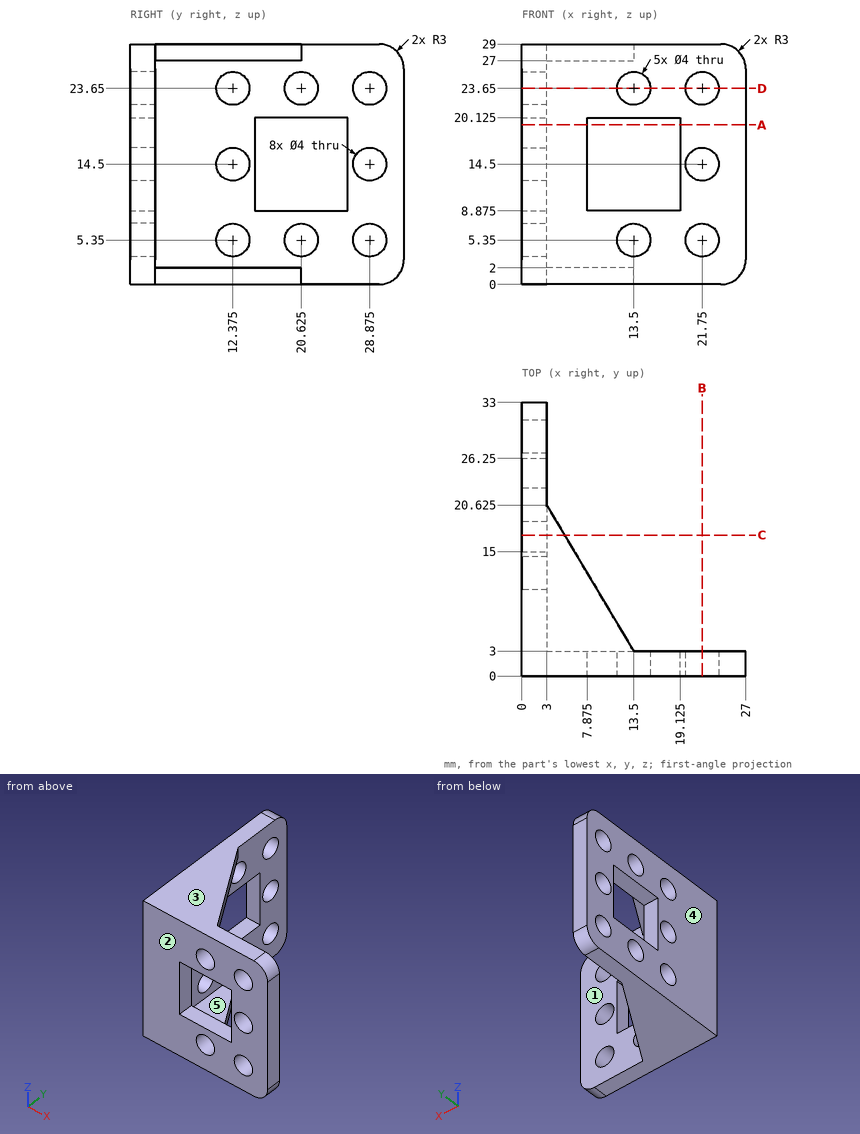
Check sheet for the drawn part. Datum: minimum x, y, z corner. Units: mm. A direction names the side the tool comes from. Round coordinates to 2 decimals unless told otherwise and drop trailing zeros. Loops run counter-clockwise (first coordinate to the right, second up) from the corner with the lowest first, then second, coordinate; pieces in that order, holes last. Notation, with made-up numbers: (24.5, -22) - (42.5, -22) arc R10 cw to (42.5, -16) - close; hole circle Ø2 at (-34.5, 42.25). An arc over 180 degrees is marked (long way). Answer as a JSON object with one key per item and string values. Group by question number.
Q1. Mould release check, pull along Z, two halves, no side actions. Record for the marked faces 3, 4 and 5: released by +Z, released by -Z, zero draft, split by the parting line, or undercut.
Q2. Sectioned sample at D-D, the plane z = 23.65. Enter the section's corners in (x, y) (3 decimals), plus the area to 3 significant figures.
Q3. Sectioned sample at A-A, the plane z = 19.25. Enter the section's corners in (x, y) (3 decimals), plus the area to 4 significant figures.
Q4. Sectioned sample at C-C, the plane y = 17. Enter the section's corners in (x, z) (3 decimals), plus the area to 3 significant figures.
Q5. Scan lines: line 1 along Z through (x, y) = (21.75, 2.2); line 2 along Y through (x, z) = (2.05, 23.65) (3 decimals); line 3 along Z through (x, y) = (13.5, 1.9) (3 decimals). Record each from-to range of solid material in increasing order. Write a range as [from, to].
Q6. Gauge pin test, flat end, axial feed: P1, Ø14.5, axis at y = 11.5, z = 19, coming from the +X side. Record the tip position at first contact, or that the pin passes through.
Q7. Sectioned sample at B-B, the plane x = 21.75. Enter the section's corners in (y, z).
Q8. Set-up check for the marked faces 1 and 2: record each of +Z, -Z, +X, -X, +Y, -Y from which the full face is reachable in a straight line by a thin tool's end or side.
Solution:
{
 "1": {"face 3": "released by +Z", "face 4": "zero draft", "face 5": "undercut"},
 "2": {"outline": "(0, 0) - (11.5, 0) - (11.5, 3) - (3, 3) - (3, 10.375) - (0, 10.375) - close; (0, 14.375) - (3, 14.375) - (3, 18.625) - (0, 18.625) - close; (0, 22.625) - (3, 22.625) - (3, 26.875) - (0, 26.875) - close; (0, 30.875) - (3, 30.875) - (3, 33) - (0, 33) - close; (15.5, 0) - (19.75, 0) - (19.75, 3) - (15.5, 3) - close; (23.75, 0) - (27, 0) - (27, 3) - (23.75, 3) - close", "area": "111 mm²"},
 "3": {"outline": "(0, 0) - (7.875, 0) - (7.875, 3) - (3, 3) - (3, 15) - (0, 15) - close; (0, 26.25) - (3, 26.25) - (3, 33) - (0, 33) - close; (19.125, 0) - (27, 0) - (27, 3) - (19.125, 3) - close", "area": "103.5 mm²"},
 "4": {"outline": "(0, 0) - (5.16, 0) - (5.16, 2) - (3, 2) - (3, 8.875) - (0, 8.875) - close; (0, 20.125) - (3, 20.125) - (3, 27) - (5.16, 27) - (5.16, 29) - (0, 29) - close", "area": "61.9 mm²"},
 "5": {"line 1": "z = [0, 3.35], [7.35, 12.5], [16.5, 21.65], [25.65, 29]", "line 2": "y = [0, 10.375], [14.375, 18.625], [22.625, 26.875], [30.875, 33]", "line 3": "z = [0, 3.35], [7.35, 8.875], [20.125, 21.65], [25.65, 29]"},
 "6": {"P1": "stops at x = 3"},
 "7": {"outline": "(0, 0) - (3, 0) - (3, 3.35) - (0, 3.35) - close; (0, 7.35) - (3, 7.35) - (3, 12.5) - (0, 12.5) - close; (0, 16.5) - (3, 16.5) - (3, 21.65) - (0, 21.65) - close; (0, 25.65) - (3, 25.65) - (3, 29) - (0, 29) - close"},
 "8": {"face 1": "+X, +Y", "face 2": "+Z, -Z, +X, -X, -Y"}
}
